The listing builds one solid part. Answer for the finished solid, in the listing's coordinates (mm). A direction names the side the tool comes from. Coordinates: 2 decimals unless noted, no trailing zeros. Order: outer loops, then holes, each group sorted by start corner. A loop starts at its lowest first (then second) coordinate and runs counter-clockwise, first axis right, second up. Notation, with made-up numbers: (26.5, 53.5) -> (48.5, 53.5) arc R36 ccw to (48.5, 88.5) -> close; hole circle Ø9 at (-33.5, 76). An arc over 180 degrees is marked (long way). Answer in a Markdown table with one row per item.
```python
from build123d import *

# Parameters (mm, degrees)
SKETCH_1_W                       = 65.418154724
SKETCH_1_H                       = 264.733197448
SM_BASE_FLANGE_1_DEPTH           = 3
SM_EDGE_FLANGE_1_STRIP_W         = 13.48
SM_EDGE_FLANGE_1_STRIP_H         = 3
SM_EDGE_FLANGE_1_STRIP_CUT_DEPTH = 264.733197448
SM_EDGE_FLANGE_1_DEPTH           = 264.733197448
SM_EDGE_FLANGE_1_FLAT_DEPTH      = 3
OTHER_START                      = -65.418154724
OTHER_1_DEPTH                    = 3


# Read off the part's stored shape, not the designer's step: Полость1
# Sheet-metal steps are written as plain solids
with BuildPart() as part:
    # Sketch 1 → Базовая кромка1 (new body)
    with BuildSketch(Plane(origin=(0, 0, 0), x_dir=(1, 0, 0), z_dir=(0, 1, 0))):
        with Locations((-32.709077362, 29.633401276)):
            Rectangle(SKETCH_1_W, SKETCH_1_H)
    extrude(amount=SM_BASE_FLANGE_1_DEPTH)

    # Ребро-кромка1 strip (across the edge) → Ребро-кромка1 strip cut (cut)
    with BuildSketch(Plane(origin=(-65.418154724, 3, -162), x_dir=(1, 0, 0), z_dir=(0, 0, 1))):
        with Locations((-3, -1.5)):
            Rectangle(SM_EDGE_FLANGE_1_STRIP_W, SM_EDGE_FLANGE_1_STRIP_H)
    extrude(amount=SM_EDGE_FLANGE_1_STRIP_CUT_DEPTH, mode=Mode.SUBTRACT)

    # Ребро-кромка1 bend section (across the edge) → Ребро-кромка1 (add)
    with BuildSketch(Plane(origin=(-65.418154724, 3, -162), x_dir=(1, 0, 0), z_dir=(0, 0, 1))):
        with BuildLine():
            Line((0, 0.74), (3, 0.74))
            ThreePointArc((3, 0.74), (3.216740982, 0.216740982), (3.74, 0))
            Line((3.74, 0), (3.74, -3))
            ThreePointArc((3.74, -3), (1.095420638, -1.904579362), (0, 0.74))
        make_face()
    extrude(amount=SM_EDGE_FLANGE_1_DEPTH)

    # Ребро-кромка1 profile (on flange) → Ребро-кромка1 flat (add)
    with BuildSketch(Plane(origin=(-65.418154724, 3, 0), x_dir=(0, 0, 1), z_dir=(-1, 0, 0))):
        Polygon((-162, 0.74), (102.733197448, 0.74), (102.733197448, 42), (40.090960975, 73.22618932), (-137.247403995, 73.22618932), (-162, 42), align=None)
    extrude(amount=-SM_EDGE_FLANGE_1_FLAT_DEPTH)

    # Полость1 outline → Полость1 (cut)
    with BuildSketch(Plane.YZ.offset(OTHER_START)):
        with BuildLine():
            ThreePointArc((44.22618932, 30), (42.104868976, 29.121320344), (41.22618932, 27))
            Line((41.22618932, 27), (41.22618932, 3))
            ThreePointArc((41.22618932, 3), (42.104868976, 0.878679656), (44.22618932, 0))
            Line((44.22618932, 0), (68.22618932, 0))
            ThreePointArc((68.22618932, 0), (70.347509663, 0.878679657), (71.22618932, 3))
            Line((71.22618932, 3), (71.22618932, 27))
            ThreePointArc((71.22618932, 27), (70.347509663, 29.121320343), (68.22618932, 30))
            Line((68.22618932, 30), (44.22618932, 30))
        make_face()
        with BuildLine():
            ThreePointArc((44.22618932, -100), (42.104868976, -100.878679656), (41.22618932, -103))
            Line((41.22618932, -103), (41.22618932, -127))
            ThreePointArc((41.22618932, -127), (42.104868976, -129.121320344), (44.22618932, -130))
            Line((44.22618932, -130), (68.22618932, -130))
            ThreePointArc((68.22618932, -130), (70.347509663, -129.121320344), (71.22618932, -127))
            Line((71.22618932, -127), (71.22618932, -103))
            ThreePointArc((71.22618932, -103), (70.347509663, -100.878679656), (68.22618932, -100))
            Line((68.22618932, -100), (44.22618932, -100))
        make_face()
    extrude(amount=OTHER_1_DEPTH, mode=Mode.SUBTRACT)

    # Зеркальное отражение1: part across plane


with BuildPart() as part_1:
    add(part.part)
    add(part.part.mirror(Plane(origin=(0, 3, -162), x_dir=(0, 0, 1), z_dir=(-1, 0, 0))))


solid = part_1.part
```
(1) Find the intervals of material crossed by line 1 along X through (y, z) = (33, -144); line 2 along Y through (x, z) = (-35.5, -101.5), in increasing order. Write a range as from..to.
Check values:
| item | result |
|---|---|
| line 1 | -65.42..-62.42, 62.42..65.42 |
| line 2 | 0..3 |
(2) Which of the six approach directions +Z, -Z, +X, -X, +Y, -Y give full straight-line access (tool end or side, diameter ignored) to faces 4 (the flat face through (-62.418, 40, -31)), 5 (the flat face through (-63.94, 60.83, -149.45))?
Check values:
| item | result |
|---|---|
| face 4 | +Z, -Z, +Y |
| face 5 | -Z, +X, -X, +Y |
(3) Flat-ended cylindrical pins translate along their axes: pin 1 (3.5 mm diameter, centred on x = -64, y = 52, fed in from -Z); pin 2 (2.5 mm diameter, centred on x = -64, z = -115, fed in from -Y); pin 3 (2.5 mm diameter, centred on x = -64, y = 57.5, fed in from -Z). Find the tip coordinate at first contact, or state that the pin passes through.
Check values:
| item | result |
|---|---|
| pin 1 | z = -157.84 |
| pin 2 | y = 0.16 |
| pin 3 | z = -153.08 |
(4) A cutting plane is placed at D-D, the plane z = -10. Determine the outline of the cut face in (x, y), then the cut area to 3 significant figures.
Check values:
| item | result |
|---|---|
| outline | (-65.42, 3.74) arc R3.74 ccw to (-61.68, 0) -> (61.68, 0) arc R3.74 ccw to (65.42, 3.74) -> (65.42, 76.23) -> (62.42, 76.23) -> (62.42, 3.74) arc R0.74 cw to (61.68, 3) -> (-61.68, 3) arc R0.74 cw to (-62.42, 3.74) -> (-62.42, 76.23) -> (-65.42, 76.23) -> close |
| area | 826 mm² |
(5) For a pull along X with two mould halves and no side action, classify faces 1 (the flat face through (63.94, 60.83, -149.45)), 2 (the flat face through (1, 3, -31)), 3 (the flat face through (-65.418, 40, -31)) as released by +X, released by -X, zero draft, split by the parting line, or undercut.
Check values:
| item | result |
|---|---|
| face 1 | zero draft |
| face 2 | undercut |
| face 3 | released by -X |
(6) A cutting plane is placed at A-A, the plane y = 30. Determine the outline of the cut face in (x, z).
Check values:
| item | result |
|---|---|
| outline | (-65.42, -162) -> (-62.42, -162) -> (-62.42, 102.73) -> (-65.42, 102.73) -> close; (62.42, -162) -> (65.42, -162) -> (65.42, 102.73) -> (62.42, 102.73) -> close |
(7) A cutting plane is placed at B-B, the plane z = -112.5. Determine the outline of the cut face in (x, y).
Check values:
| item | result |
|---|---|
| outline | (-65.42, 3.74) arc R3.74 ccw to (-61.68, 0) -> (61.68, 0) arc R3.74 ccw to (65.42, 3.74) -> (65.42, 41.23) -> (62.42, 41.23) -> (62.42, 3.74) arc R0.74 cw to (61.68, 3) -> (-61.68, 3) arc R0.74 cw to (-62.42, 3.74) -> (-62.42, 41.23) -> (-65.42, 41.23) -> close; (-65.42, 71.23) -> (-62.42, 71.23) -> (-62.42, 76.23) -> (-65.42, 76.23) -> close; (62.42, 71.23) -> (65.42, 71.23) -> (65.42, 76.23) -> (62.42, 76.23) -> close |
(8) A cutting plane is placed at C-C, the plane y = 59.5. Determine the outline of the cut face in (x, z), then the cut area to 3 significant figures.
Check values:
| item | result |
|---|---|
| outline | (-65.42, -150.51) -> (-62.42, -150.51) -> (-62.42, -130) -> (-65.42, -130) -> close; (-65.42, -100) -> (-62.42, -100) -> (-62.42, 0) -> (-65.42, 0) -> close; (-65.42, 30) -> (-62.42, 30) -> (-62.42, 73.65) -> (-65.42, 73.65) -> close; (62.42, -150.51) -> (65.42, -150.51) -> (65.42, -130) -> (62.42, -130) -> close; (62.42, -100) -> (65.42, -100) -> (65.42, 0) -> (62.42, 0) -> close; (62.42, 30) -> (65.42, 30) -> (65.42, 73.65) -> (62.42, 73.65) -> close |
| area | 985 mm² |
